```python
from build123d import *
from build123d.topology import SkipClean

# Parameters (mm, degrees)
ESBO_O1_R                  = 0.5
RESSALTO_EXTRUS_O1_DEPTH   = 0.2
FILETE1_R                  = 0.15
FILETE2_R                  = 0.15
ESBO_O6_W                  = 10
ESBO_O6_H                  = 0.2
RESSALTO_EXTRUS_O2_DEPTH   = 0.5
RESSALTO_EXTRUS_O3_DEPTH   = 10
CORTE_EXTRUS_O1_DEPTH      = 10
CORTE_EXTRUS_O2_DEPTH      = 10
CORTE_EXTRUS_O2_DEPTH_BACK = 10
ESBO_O9_W                  = 2.5
ESBO_O9_H                  = 2


with BuildPart() as part:
    # Esboço1 → Ressalto-extrusão1 (new body)
    with BuildSketch(Plane.XY):
        with BuildLine():
            Line((-19.847807635, 8.186498983), (-9.847807635, 8.186498983))
            Line((-9.847807635, 8.186498983), (-13.047807635, -5.813501017))
            ThreePointArc((-13.047807635, -5.813501017), (-15.047807635, -7.813501017), (-17.047807635, -5.813501017))
            Line((-17.047807635, -5.813501017), (-19.847807635, 8.186498983))
        make_face()
        with Locations((-12.847807635, 4.283271461)):
            Circle(ESBO_O1_R, mode=Mode.SUBTRACT)
        with Locations((-16.847807635, 5.652628285)):
            Circle(ESBO_O1_R, mode=Mode.SUBTRACT)
        with Locations((-15.047807635, -5.813501017)):
            Circle(ESBO_O1_R, mode=Mode.SUBTRACT)
    extrude(amount=RESSALTO_EXTRUS_O1_DEPTH)

    # Filete1
    filete1_edges = [part.edges().sort_by_distance(p)[0] for p in [
        (-17.347807635, 5.652628285, 0),
        (-13.347807635, 4.283271461, 0),
        (-15.547807635, -5.813501017, 0.2),
    ]]
    fillet(filete1_edges, radius=FILETE1_R)

    # Filete2
    # the kernel refuses this fillet: 0.15 mm, written as the material it takes off along each edge
    with BuildSketch(Plane(origin=(-15.047807635, -5.813501017, 0), x_dir=(1, 0, 0), z_dir=(0, -1, 0))) as filete2_piece_1:
        with BuildLine():
            CenterArc((0.611803399, 0.15), FILETE2_R, 221.810314896, 48.189685104)
            Line((0.5, 0.05), (0.497763932, 0.048))
            ThreePointArc((0.497763932, 0.048), (0.497, 0.025), (0.497, 0))
            Line((0.497, 0), (0.5, -0.003))
            Line((0.5, -0.003), (0.611803399, -0.003))
            Line((0.611803399, -0.003), (0.611803399, 0))
        make_face()
    revolve(axis=Axis((-15.047807635, -5.813501017, 0), (0, 0, 1)), mode=Mode.SUBTRACT)
    with BuildSketch(Plane(origin=(-12.847807635, 4.283271461, 0.2), x_dir=(1, 0, 0), z_dir=(0, -1, 0))) as filete2_piece_2:
        with BuildLine():
            CenterArc((0.611803399, -0.15), FILETE2_R, 90, 48.189685104)
            Line((0.611803399, 0), (0.611803399, 0.003))
            Line((0.611803399, 0.003), (0.5, 0.003))
            Line((0.5, 0.003), (0.497, 0))
            ThreePointArc((0.497, 0), (0.497, -0.025), (0.497763932, -0.048))
            Line((0.497763932, -0.048), (0.5, -0.05))
        make_face()
    revolve(axis=Axis((-12.847807635, 4.283271461, 0.2), (0, 0, 1)), mode=Mode.SUBTRACT)
    with BuildSketch(Plane(origin=(-16.847807635, 5.652628285, 0.2), x_dir=(1, 0, 0), z_dir=(0, -1, 0))) as filete2_piece_3:
        with BuildLine():
            CenterArc((0.611803399, -0.15), FILETE2_R, 90, 48.189685104)
            Line((0.5, -0.05), (0.497763932, -0.048))
            ThreePointArc((0.497763932, -0.048), (0.497, -0.025), (0.497, 0))
            Line((0.497, 0), (0.5, 0.003))
            Line((0.5, 0.003), (0.611803399, 0.003))
            Line((0.611803399, 0.003), (0.611803399, 0))
        make_face()
    revolve(axis=Axis((-16.847807635, 5.652628285, 0.2), (0, 0, 1)), mode=Mode.SUBTRACT)

    # Esboço6 → Ressalto-extrusão2 (add)
    with BuildSketch(Plane(origin=(0, 8.186498983, 0), x_dir=(1, 0, 0), z_dir=(0, 1, 0))):
        with Locations((-14.847807635, -0.1)):
            Rectangle(ESBO_O6_W, ESBO_O6_H)
    extrude(amount=RESSALTO_EXTRUS_O2_DEPTH)

    # Esboço7 → Ressalto-extrusão3 (add)
    with BuildSketch(Plane(origin=(-9.847807635, 0, 0), x_dir=(0, 0, -1), z_dir=(1, 0, 0))):
        with BuildLine():
            ThreePointArc((0.35, 8.686498983), (-0.380624304, 9.038280165), (-0.2, 8.247750764))
            Line((-0.2, 8.247750764), (-0.2, 8.457370198))
            ThreePointArc((-0.2, 8.457370198), (-0.236930639, 8.89566399), (0.15, 8.686498983))
            ThreePointArc((0.15, 8.686498983), (0.109165007, 8.549568344), (0, 8.457370198))
            Line((0, 8.457370198), (0, 8.247750764))
            ThreePointArc((0, 8.247750764), (0.251781182, 8.405874679), (0.35, 8.686498983))
        make_face()
        with BuildLine():
            Line((-0.2, 8.457370198), (-0.2, 8.247750764))
            ThreePointArc((-0.2, 8.247750764), (-0.1, 8.236498983), (0, 8.247750764))
            Line((0, 8.247750764), (0, 8.457370198))
            ThreePointArc((0, 8.457370198), (-0.1, 8.436498983), (-0.2, 8.457370198))
        make_face()
    extrude(amount=-RESSALTO_EXTRUS_O3_DEPTH)

    # Esboço8 → Corte-extrusão1 (cut)
    with SkipClean():  # the faces are left unmerged after this step: merging them gives an invalid solid
        with BuildSketch(Plane(origin=(-9.847807635, 0, 0), x_dir=(0, 0, -1), z_dir=(1, 0, 0))):
            with BuildLine():
                ThreePointArc((-0.2, 8.457370198), (-0.1, 8.936498983), (0, 8.457370198))
                Line((0, 8.457370198), (0, 8.686498983))
                Line((0, 8.686498983), (-0.2, 8.686498983))
                Line((-0.2, 8.686498983), (-0.2, 8.457370198))
            make_face()
            with BuildLine():
                Line((0, 8.686498983), (0, 8.457370198))
                ThreePointArc((0, 8.457370198), (0.109165007, 8.549568344), (0.15, 8.686498983))
                ThreePointArc((0.15, 8.686498983), (-0.236930639, 8.89566399), (-0.2, 8.457370198))
                Line((-0.2, 8.457370198), (-0.2, 8.686498983))
                Line((-0.2, 8.686498983), (0, 8.686498983))
            make_face()
            with BuildLine():
                ThreePointArc((-0.2, 8.457370198), (-0.1, 8.436498983), (0, 8.457370198))
                Line((0, 8.457370198), (0, 8.686498983))
                Line((0, 8.686498983), (-0.2, 8.686498983))
                Line((-0.2, 8.686498983), (-0.2, 8.457370198))
            make_face()
        extrude(amount=-CORTE_EXTRUS_O1_DEPTH, mode=Mode.SUBTRACT)

    # Esboço9 → Corte-extrusão2 (cut, two sides: drawn at the far end of the back side and taken through both)
    with BuildSketch(Plane(origin=(0, 0, 0), x_dir=(-1, 0, 0), z_dir=(0, 0, -1)).offset(-CORTE_EXTRUS_O2_DEPTH_BACK)):
        with Locations((11.097807635, 9.186498983)):
            Rectangle(ESBO_O9_W, ESBO_O9_H)
        with Locations((18.597807635, 9.186498983)):
            Rectangle(ESBO_O9_W, ESBO_O9_H)
    extrude(amount=CORTE_EXTRUS_O2_DEPTH + CORTE_EXTRUS_O2_DEPTH_BACK, mode=Mode.SUBTRACT)


solid = part.part
```
Model file for the job. Use its own axes, mm. A direction names the side the tool comes from. Coordinates: 2 decimals unless noted, no trailing zeros. Order: outer loops, then holes, each group sorted by start corner. A loop starts at its lowest first (then second) coordinate and runs counter-clockwise, first axis right, second up. Notation, with made-up numbers: M -26,-13 L 8,-13 A30 ccw 8,24 Z; hole C -24.75,60 d2. An arc over 180 degrees is marked long. Answer as CSV lines item,"result".
(1) Wall check: line 1 along Z through (x, y) = (-10.5, 6); line 2 along X through (y, z) = (-5.5, 0.1); line 3 along Y through (x, z) = (-16, 0.3). Give the ranges that are in metal, low to high.
Geometry says:
line 1,"z = 0 to 0.2"
line 2,"x = -17.11 to -15.45, -14.65 to -12.98"
line 3,"y = 8.28 to 8.54, 8.84 to 9.09"
(2) Flat gauge pin, fed straight in: pin 1 (3 mm diameter, centred on x = -16, y = -3.5, fed in from -Z). Where does the tip first touch, or does it go through?
Geometry says:
pin 1,"stops at z = 0"
(3) 3-axis set-ups, long thin cutter, end or side, ignore diameter. For faces 1 (the flat face through (-15, 2, 0.2)), 2 (the flat face through (-15, 2, 0)): which of +Z, -Z, +X, -X, +Y, -Y reach the whole face in a straight line?
Geometry says:
face 1,"+Z, +X, -X, -Y"
face 2,"-Z, +X, -X, -Y"
(4) Band-saw the part on A-A, the plane x = -14. List the corners of the cut face in (y, z), then the cut area to 3 significant figures.
Geometry says:
outline,"M -7.52,0 L 8.25,0 A0.45 ccw long 8.25,0.2 L -7.52,0.2 Z; hole C 8.69,0.1 d0.5"
area,"3.59 mm2"
(5) Band-saw the part on C-C, the plane x = -11.5. List the corners of the cut face in (y, z).
Geometry says:
outline,"M 0.96,0 L 8.19,0 L 8.19,0.2 L 0.96,0.2 Z"
(6) Band-saw the part on B-B, the plane y = -4.5. List the corners of the cut face in (x, z).
Geometry says:
outline,"M -17.31,0 L -12.75,0 L -12.75,0.2 L -17.31,0.2 Z"
